Source: CAD feature listing. Evaluate the final solid. Frame: model axes, mm. Face numbers are marked on the shaded views. A direction names the side the tool comes from. Give positions to 0.01 mm unless a question says otherwise; leave off trailing zeros. Loops run counter-clockwise (first coordinate to the right, second up) from the corner with the lowest first, then second, coordinate; pieces in that order, holes last. Notation, with made-up numbers: M 35.25,-13.75 L 78.25,-13.75 A23 cw 78.25,-5.75 Z; hole C 66,5.25 d11. An arc over 180 degrees is marked long. Answer in a Markdown table with one row per item.
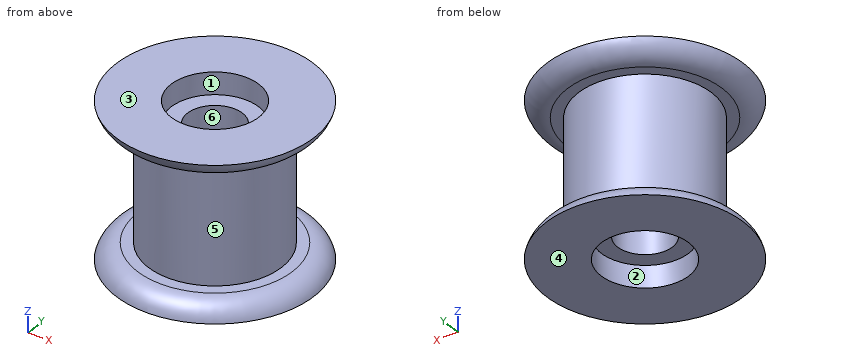
```python
from build123d import *

# Parameters (mm, degrees)
FILLET1_R          = 2
SKETCH2_R          = 4
CUT_EXTRUDE2_DEPTH = 2
SKETCH4_R          = 2.5
CUT_EXTRUDE3_DEPTH = 10


with BuildPart() as part:
    # Sketch1 → Revolve1 (revolve)
    with BuildSketch(Plane(origin=(0, 0, 0), x_dir=(1, 0, 0), z_dir=(0, 1, 0)), mode=Mode.PRIVATE) as revolve1_sk:
        Polygon((0, 0), (9, 0), (9, -1.5), (6.07, -1.5), (6.07, -12.5), (9, -12.5), (9, -14), (0, -14), align=None)
    revolve(revolve1_sk.sketch.rotate(Axis((0, 0, -9.941176471), (0, 0, 1)), 180), axis=Axis((0, 0, -9.941176471), (0, 0, 1)))

    # Fillet1
    # the kernel refuses this fillet: 2 mm, written as the material it takes off along each edge
    with BuildSketch(Plane(origin=(0, 0, 12.5), x_dir=(-1, 0, 0), z_dir=(0, 1, 0))) as fillet1_piece_1:
        with BuildLine():
            CenterArc((7.063508327, 2), FILLET1_R, 270, 75.522487814)
            Line((9, 1.5), (9.038729833, 1.49))
            ThreePointArc((9.038729833, 1.49), (9.04, 0.75), (9.04, 0))
            Line((9.04, 0), (9, -0.04))
            Line((9, -0.04), (7.063508327, -0.04))
            Line((7.063508327, -0.04), (7.063508327, 0))
        make_face()
    revolve(axis=Axis((0, 0, 12.5), (0, 0, 1)), mode=Mode.SUBTRACT)
    with BuildSketch(Plane(origin=(0, 0, 1.5), x_dir=(-1, 0, 0), z_dir=(0, 1, 0))) as fillet1_piece_2:
        with BuildLine():
            CenterArc((7.063508327, -2), FILLET1_R, 14.477512186, 75.522487814)
            Line((7.063508327, 0), (7.063508327, 0.04))
            Line((7.063508327, 0.04), (9, 0.04))
            Line((9, 0.04), (9.04, 0))
            ThreePointArc((9.04, 0), (9.04, -0.75), (9.038729833, -1.49))
            Line((9.038729833, -1.49), (9, -1.5))
        make_face()
    revolve(axis=Axis((0, 0, 1.5), (0, 0, 1)), mode=Mode.SUBTRACT)

    # Sketch2 → Cut-Extrude2 (cut)
    with BuildSketch(Plane(origin=(0, 0, 0), x_dir=(-1, 0, 0), z_dir=(0, 0, -1))):
        Circle(SKETCH2_R)
    cut_extrude2 = extrude(amount=-CUT_EXTRUDE2_DEPTH, mode=Mode.SUBTRACT)

    # Mirror1: Cut-Extrude2 across plane
    add(cut_extrude2.mirror(Plane(origin=(0, 0, 7), x_dir=(1, 0, 0), z_dir=(0, 0, -1))), mode=Mode.SUBTRACT)

    # Sketch4 → Cut-Extrude3 (cut)
    with BuildSketch(Plane.XY.offset(12)):
        Circle(SKETCH4_R)
    extrude(amount=-CUT_EXTRUDE3_DEPTH, mode=Mode.SUBTRACT)


solid = part.part
```
Q1. Mould query, pull axis Y, two halves, no side actions, for the marked faces 4, 5 and 6. Classes: +Y half, -Y half, draft (parallel to the pull), parting line (faces both ways), or undercut.
Values follow:
| item | result |
|---|---|
| face 4 | draft |
| face 5 | parting line |
| face 6 | undercut |
Q2. Contact query for flat-ended pins moving along their axis: pin 1 Ø6.5 at (x, y) = (0, 0) entering from -Z; pin 2 Ø6 at (x, y) = (0, 0) entering from +Z; pin 3 Ø6 at (x, z) = (-5, 5) entering from -Y. Output: stop coordinate, or through.
Values follow:
| item | result |
|---|---|
| pin 1 | z = 2 |
| pin 2 | z = 12 |
| pin 3 | y = -5.73 |
Q3. Section query C-C (z = 8). Output: boundary loops of the cut face in (x, y), plus the area to 3 significant figures.
Values follow:
| item | result |
|---|---|
| outline | C 0,0 d12.14; hole C 0,0 d5 |
| area | 96.1 mm^2 |
Q4. Reachability of the marked faces 1, 2 and 3 from +Z, -Z, +X, -X, +Y, -Y: full face, straight path, thin tool, end or side. Return the list, or none.
Values follow:
| item | result |
|---|---|
| face 1 | +Z |
| face 2 | -Z |
| face 3 | +Z, +X, -X, +Y, -Y |
Q5. Ray query, probe 1 along Z at (x, y) = (0.75, -7); probe 2 along Y at (x, z) = (0, 5); probe 3 along Y at (x, z) = (0, 1.6). Return the intervals inside material, ascending. Write a range as from..to.
Values follow:
| item | result |
|---|---|
| probe 1 | 0..1.5, 12.5..14 |
| probe 2 | -6.07..-2.5, 2.5..6.07 |
| probe 3 | -6.07..-4, 4..6.07 |
Q6. Section query A-A (x = 0). Output: boundary loops of the cut face in (y, z), plus the area to 3 significant figures.
Values follow:
| item | result |
|---|---|
| outline | M -9,0 L -4,0 L -4,2 L -2.5,2 L -2.5,12 L -4,12 L -4,14 L -9,14 A2 ccw -7.06,12.5 L -6.07,12.5 L -6.07,1.5 L -7.06,1.5 A2 ccw Z; M 2.5,2 L 4,2 L 4,0 L 9,0 A2 ccw 7.06,1.5 L 6.07,1.5 L 6.07,12.5 L 7.06,12.5 A2 ccw 9,14 L 4,14 L 4,12 L 2.5,12 Z |
| area | 103 mm^2 |
